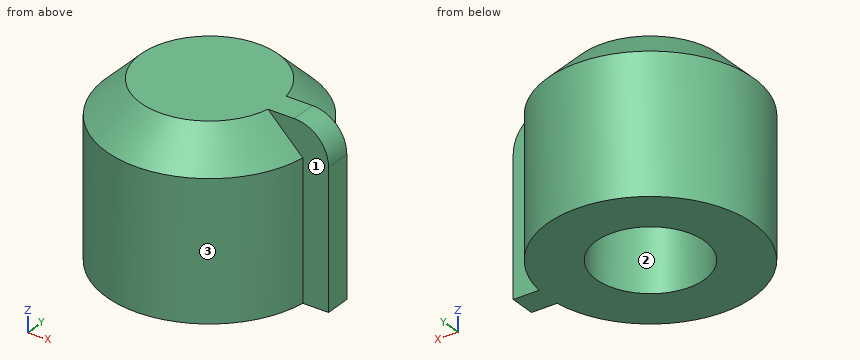
```python
from build123d import *

# Parameters (mm, degrees)
SKETCH_R     = 6
PAD_DEPTH    = 10
SKETCH001_R  = 3.15
POCKET_DEPTH = 8
PAD001_DEPTH = 1
SKETCH003_W  = 1.5
SKETCH003_H  = 1.5
PAD002_DEPTH = 10
CHAMFER_SIZE = 2
FILLET_R     = 2


with BuildPart() as part:
    # Sketch → Pad (new body)
    with BuildSketch(Plane.XY):
        Circle(SKETCH_R)
    extrude(amount=PAD_DEPTH)

    # Sketch001 (on Face2 of Pad) → Pocket (cut)
    with BuildSketch(Plane(origin=(0, 0, 0), x_dir=(1, 0, 0), z_dir=(0, 0, -1))):
        Circle(SKETCH001_R)
    extrude(amount=-POCKET_DEPTH, mode=Mode.SUBTRACT)

    # Sketch002 (on Face5 of Pocket) → Pad001 (join)
    with BuildSketch(Plane(origin=(0, 0, 8), x_dir=(1, 0, 0), z_dir=(0, 0, -1))):
        with BuildLine():
            Line((-3.071238, 0.7), (3.071238, 0.7))
            ThreePointArc((3.059412, -0.75), (3.149895, -0.02569), (3.071238, 0.7))
            Line((3.059412, -0.75), (-3.059412, -0.75))
            ThreePointArc((-3.071238, 0.7), (-3.149895, -0.02569), (-3.059412, -0.75))
        make_face()
    extrude(amount=PAD001_DEPTH)

    # Sketch003 (on Face2 of Pad001) → Pad002 (join)
    with BuildSketch(Plane(origin=(0, 0, 0), x_dir=(1, 0, 0), z_dir=(0, 0, -1))):
        with Locations((6.70294, 0)):
            Rectangle(SKETCH003_W, SKETCH003_H)
    extrude(amount=-PAD002_DEPTH)

    # Chamfer
    chamfer_edges = [part.edges().sort_by_distance(p)[0] for p in [
        (-6, 0, 10),
    ]]
    chamfer(chamfer_edges, length=CHAMFER_SIZE)

    # Fillet
    fillet_edges = [part.edges().sort_by_distance(p)[0] for p in [
        (7.45294, 0, 10),
    ]]
    fillet(fillet_edges, radius=FILLET_R)


solid = part.part
```
Verification items for the finished model (mm, model axes). Face numbers are marked on the shaded views. Coordinates: 2 decimals unless noted, no trailing zeros. Loops run counter-clockwise (first coordinate to the right, second up) from the corner with the lowest first, then second, coordinate; pieces in that order, holes last. Notation, with made-up numbers: (-33.75, -3) -> (-0.75, -3) arc R20 cw to (-0.75, 24) -> close; hole circle Ø8 at (25.25, 23.25). An arc over 180 degrees is marked (long way). Answer in a Markdown table with one row per item. Add a question column.
1. Section check A-A, the plane x = 0. Enter the section's corners in (y, z).
2. Section check B-B, the plane y = 0. Enter the section's corners in (x, z).
3. Section check D-D, the plane z = 1.5. Enter the section's corners in (x, y).
4. Section check C-C, the plane z = 7.5. Enter the section's corners in (x, y), then the cut area to 3 significant figures.
5. Material ranges on probe 1 along Y at (x, z) = (0, 3.5); probe 2 along Y at (x, z) = (1.25, 7.25); probe 3 along Z at (x, y) = (-0.5, 0), recorded low to high. Write a range as [from, to].
6. Depth check by flat-ended pin: P1, Ø1.8, axis at x = 5, z = 4, coming from the -Y side; P2, Ø1.5, axis at x = 1, y = 0.5, coming from the -Z side; P3, Ø1.5, axis at x = 5.5, z = 1.5, coming from the -Y side. Enter the tip coordinate at first touch or a pass-through.
7. Draft check along X on the marked faces 1, 2 and 3. Enter one of: +X half, -X half, draft (parallel to the pull), parting line (faces both ways), or undercut.
Derived:
| question | item | result |
|---|---|---|
| 1 | outline | (-6, 0) -> (-3.15, 0) -> (-3.15, 8) -> (-0.7, 8) -> (-0.7, 7) -> (0.75, 7) -> (0.75, 8) -> (3.15, 8) -> (3.15, 0) -> (6, 0) -> (6, 8) -> (4, 10) -> (-4, 10) -> (-6, 8) -> close |
| 2 | outline | (-6, 0) -> (-3.15, 0) -> (-3.15, 7) -> (3.15, 7) -> (3.15, 0) -> (7.45, 0) -> (7.45, 8) arc R2 ccw to (5.45, 10) -> (-4, 10) -> (-6, 8) -> close |
| 3 | outline | (5.95, -0.75) -> (7.45, -0.75) -> (7.45, 0.75) -> (5.95, 0.75) arc R6 ccw (long way) to start; hole circle Ø6.3 at (0, 0) |
| 4 | outline | (5.95, -0.75) -> (7.45, -0.75) -> (7.45, 0.75) -> (5.95, 0.75) arc R6 ccw (long way) to start; hole (-3.07, -0.7) arc R3.15 ccw to (3.07, -0.7) -> close; hole (-3.06, 0.75) -> (3.06, 0.75) arc R3.15 ccw to start |
| 4 | area | 93.2 mm² |
| 5 | probe 1 | y = [-6, -3.15], [3.15, 6] |
| 5 | probe 2 | y = [-5.87, -2.89], [-0.7, 0.75], [2.89, 5.87] |
| 5 | probe 3 | z = [7, 10] |
| 6 | P1 | stops at y = -4.38 |
| 6 | P2 | stops at z = 7 |
| 6 | P3 | stops at y = -3.67 |
| 7 | face 1 | draft |
| 7 | face 2 | undercut |
| 7 | face 3 | parting line |
